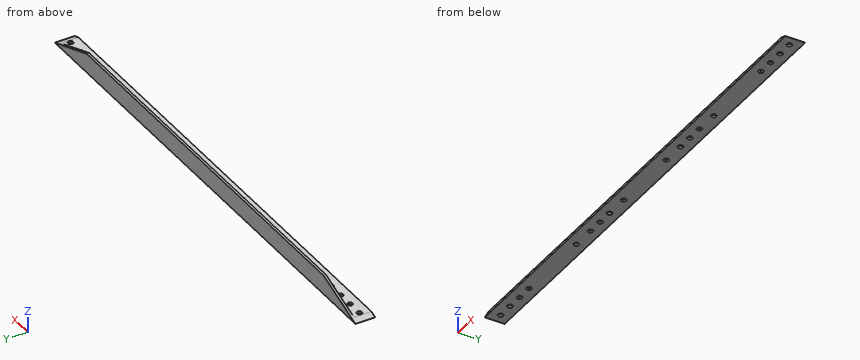
from build123d import *

# Parameters (mm, degrees)
SKETCH_1_W          = 2540
SKETCH_1_H          = 100
SKETCH_1_R          = 13
EXTRUDE_525_DEPTH   = 12
SKETCH_2_W          = 2540
SKETCH_2_H          = 12
EXTRUDE_1_DEPTH     = 86
CUT_EXTRUDE_1_DEPTH = 1278.694799238


with BuildPart() as part:
    # 草图1 → Extrude 525 (new body)
    with BuildSketch(Plane.XY):
        Rectangle(SKETCH_1_W, SKETCH_1_H)
        with Locations((1220, 0)):
            Circle(SKETCH_1_R, mode=Mode.SUBTRACT)
        with Locations((1140, 0)):
            Circle(SKETCH_1_R, mode=Mode.SUBTRACT)
        with Locations((1060, 0)):
            Circle(SKETCH_1_R, mode=Mode.SUBTRACT)
        with Locations((980, 0)):
            Circle(SKETCH_1_R, mode=Mode.SUBTRACT)
        with Locations((580, 0)):
            Circle(SKETCH_1_R, mode=Mode.SUBTRACT)
        with Locations((460, 0)):
            Circle(SKETCH_1_R, mode=Mode.SUBTRACT)
        with Locations((380, 0)):
            Circle(SKETCH_1_R, mode=Mode.SUBTRACT)
        with Locations((300, 0)):
            Circle(SKETCH_1_R, mode=Mode.SUBTRACT)
        with Locations((180, 0)):
            Circle(SKETCH_1_R, mode=Mode.SUBTRACT)
        with Locations(Location((-180, 0, 0), (0, 0, 180))):
            Circle(SKETCH_1_R, mode=Mode.SUBTRACT)
        with Locations(Location((-300, 0, 0), (0, 0, 180))):
            Circle(SKETCH_1_R, mode=Mode.SUBTRACT)
        with Locations(Location((-380, 0, 0), (0, 0, 180))):
            Circle(SKETCH_1_R, mode=Mode.SUBTRACT)
        with Locations(Location((-460, 0, 0), (0, 0, 180))):
            Circle(SKETCH_1_R, mode=Mode.SUBTRACT)
        with Locations(Location((-580, 0, 0), (0, 0, 180))):
            Circle(SKETCH_1_R, mode=Mode.SUBTRACT)
        with Locations(Location((-980, 0, 0), (0, 0, 180))):
            Circle(SKETCH_1_R, mode=Mode.SUBTRACT)
        with Locations(Location((-1060, 0, 0), (0, 0, 180))):
            Circle(SKETCH_1_R, mode=Mode.SUBTRACT)
        with Locations(Location((-1140, 0, 0), (0, 0, 180))):
            Circle(SKETCH_1_R, mode=Mode.SUBTRACT)
        with Locations(Location((-1220, 0, 0), (0, 0, 180))):
            Circle(SKETCH_1_R, mode=Mode.SUBTRACT)
    extrude(amount=EXTRUDE_525_DEPTH)

    # 草图2 → 凸台-拉伸1 (add)
    with BuildSketch(Plane.XY.offset(12)):
        with Locations((0, 44)):
            Rectangle(SKETCH_2_W, SKETCH_2_H)
    extrude(amount=EXTRUDE_1_DEPTH)

    # 草图4 → 切除-拉伸1 (cut, through all)
    with BuildSketch(Plane(origin=(0, 50, 0), x_dir=(-1, 0, 0), z_dir=(0, 1, 0))):
        Polygon((-1270, 0), (-1270, 98), (-1000, 98), align=None)
        Polygon((1270, 0), (1000, 98), (1270, 98), align=None)
    extrude(amount=-CUT_EXTRUDE_1_DEPTH, mode=Mode.SUBTRACT)


solid = part.part
Verification items for the finished model (mm, model axes). Give positions to 0.01 mm unless a question says otherwise; leave off trailing zeros. Order: outer loops, then holes, each group sorted by start corner. A loop starts at its lowest first (then second) coordinate and runs counter-clockwise, first axis right, second up. Notation, with made-up numbers: M 3,19 L 61,19 A15 cw 61,27 Z; hole C 44.25,31 d2. An arc over 180 degrees is marked long. Answer as a JSON object with one key per item and string values. Group by question number.
1) Depth check by flat-ended pin: pin 1 Ø15.5 at (x, y) = (-1140, 0) entering from +Z; pin 2 Ø4 at (x, y) = (-359.5, -4) entering from +Z; pin 3 Ø5 at (x, z) = (684.5, 62.5) entering from -Y; pin 4 Ø2 at (x, y) = (-153.5, 16.5) entering from -Z. Enter the tip coordinate at first touch or a pass-through.
2) Cross-section at A-A (x = 944.5). Enter the section's corners in (y, z).
3) Scan lines: line 1 along Y through (x, z) = (-180, 6.5); line 2 along Z through (x, y) = (-1102, 31); line 3 along Y through (x, z) = (-893, 48). Record each from-to range of solid material in increasing order. Write a range as [from, to].
4) Cross-section at B-B (z = 28). Enter the section's corners in (x, y), then the cut area to 3 significant figures.
Result sheet:
{
 "1": {"pin 1": "passes through", "pin 2": "stops at z = 12", "pin 3": "stops at y = 38", "pin 4": "stops at z = 0"},
 "2": {"outline": "M -50,0 L 50,0 L 50,98 L 38,98 L 38,12 L -50,12 Z"},
 "3": {"line 1": "y = [-50, -13], [13, 50]", "line 2": "z = [0, 12]", "line 3": "y = [38, 50]"},
 "4": {"outline": "M -1192.86,38 L 1192.86,38 L 1192.86,50 L -1192.86,50 Z", "area": "28,600 mm2"}
}
